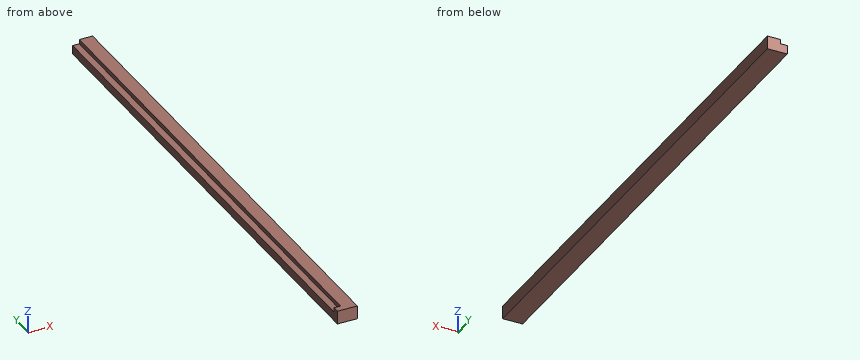
Autodesk Inventor part; units mm, degrees
ref_plane "YZ Plane" through (0, 0, 0) normal (1, 0, 0) x (0, 1, 0)
ref_plane "XZ Plane" through (0, 0, 0) normal (0, 1, 0) x (-1, 0, 0)
ref_plane "XY Plane" through (0, 0, 0) normal (0, 0, 1) x (1, 0, 0)
ref_plane "Work Plane1" through (0, 0, 0) normal (0, 0, 1) x (1, 0, 0)
sketch "Sketch1" plane through (0, 0, 0) normal (0, 0, 1) x (1, 0, 0)
  line L0 (302.4187, 990.6) -> (264.3187, 990.6)
  line L1 (264.3187, 990.6) -> (264.3188, 0)
  line L2 (264.3188, 0) -> (302.4188, 0)
  line L3 (302.4188, 0) -> (302.4187, 990.6)
  point P0 (0, 0)
  dimension "d0" = 990.6
  dimension "d2" = 38.1
extrude "Extrusion1" add sketch "Sketch1" along normal blind 25.4
sketch "Sketch3" plane through (0, 0, 25.4) normal (0, 0, 1) x (1, 0, 0)
  line L0 (264.3187, 990.6) -> (277.0187, 990.6)
  line L1 (277.0187, 990.6) -> (277.0187, 12.7)
  line L2 (277.0187, 12.7) -> (264.3187, 12.7)
  line L3 (264.3187, 12.7) -> (264.3187, 990.6)
  point P0 (0, 0)
  dimension "d10" = 12.7
  dimension "d11" = 977.9
extrude "Extrusion3" cut sketch "Sketch3" against normal blind 8.4646
equation "\"d0\" = 0.5 * signH"
equation "\"d2\" = borderW"
equation "\"d3\" = borderH"
equation "\"d10\" = panelLap"
equation "\"d11\" = 0.5 * signH - panelLap"
equation "\"d12\" = panelH + velcroH + panelHClear"
equation "\"signH\" = 1981.2"
equation "\"borderW\" = 38.1"
equation "\"borderH\" = 25.4"
equation "\"velcroH\" = 2.54"
equation "\"panelH\" = 5.1308"
equation "\"panelHClear\" = 0.79375"
equation "\"panelLap\" = 12.7"
properties part number "SideborderInverse"
Here's how the part is built. I have some questions about the finished solid (model axes, mm). Coordinates: 2 decimals unless noted, no trailing zeros. Write each loop counter-clockwise with the first axis right and the second up, starting at its lowest first coordinate (ties: lowest second). Pieces come first, ordered by that corner, then holes.
Item 1: If I drill on line 1 (Z direction, x = 267.5, y = 755.5); line 2 (X direction, y = 91.5, z = 20.5); line 3 (Y direction, x = 275.5, z = 18), over which ranges is the centre line in solid material (lowest first)?
Item 2: Will these pins go through, and if not, where does the flat tip stop? pin 1 (2.5 mm diameter, centred on y = 597, z = 21.5, fed in from -X); pin 2 (9.5 mm diameter, centred on x = 268, z = 23.5, fed in from +Y).
Item 3: I want a section at A-A on y = 519. Write out the boundary of the cut face in (x, z).
Findings below:
1. line 1: z = 0 to 16.94
1. line 2: x = 277.02 to 302.42
1. line 3: y = 0 to 12.7
2. pin 1: stops at x = 277.02
2. pin 2: stops at y = 12.7
3. outline: (264.32, 0) - (302.42, 0) - (302.42, 25.4) - (277.02, 25.4) - (277.02, 16.94) - (264.32, 16.94) - close
